Study the drawing (mm; zero at the part's minimum x, y, z) and answer. A direction names the side the tool comes from. Round coordinates to 2 decimals unless told otherwise and drop trailing zeros. Order: outer loops, then holes, each group sorted by start corner. A loop starts at its lowest first (then second) coordinate and runs counter-clockwise, first axis right, second up. Notation, with made-up numbers: (22.25, -23) - (66.25, -23) arc R23 cw to (66.25, -8) - close; hole circle Ø2 at (31, 48). An arc over 180 degrees is marked (long way). Use one line per item in the form item = value. Start each with the question number.
Q1. Which of the six approach directions +Z, -Z, +X, -X, +Y, -Y give full straight-line access (tool end or side, diameter ignored) to the marked faces 1 and 2?
Q2. For a pull along X with two mould halves and no side action, classify the marked faces 3, 4 and 5 as +X half, -X half, draft (parallel to the pull), parting line (faces both ways), or undercut.
Q3. The part is cut by section D-D on y = 14. Determine the outline of the cut face in (x, z) (1 decimal).
Q4. Given P1, Ø1, axis at y = 15, z = 0.5, coming from the -X side (1 decimal); P2, Ø1.5, axis at y = 15.5, z = 4.5, coming from the +X side; P3, Ø1.5, axis at x = 14, z = 1.5, coming from the -Y side (3 decimals), each flat-ended and moving along its own axis, determine where each tip first touches the part or whether it passes through.
Q5. Find the intervals of material crossed by line 1 (X direction, y = 16.5, z = 3); line 2 (X direction, y = 4.75, z = 0.75) (1 decimal); line 3 (Z direction, x = 4, y = 2.25), in increasing order. Write a range as [from, to].
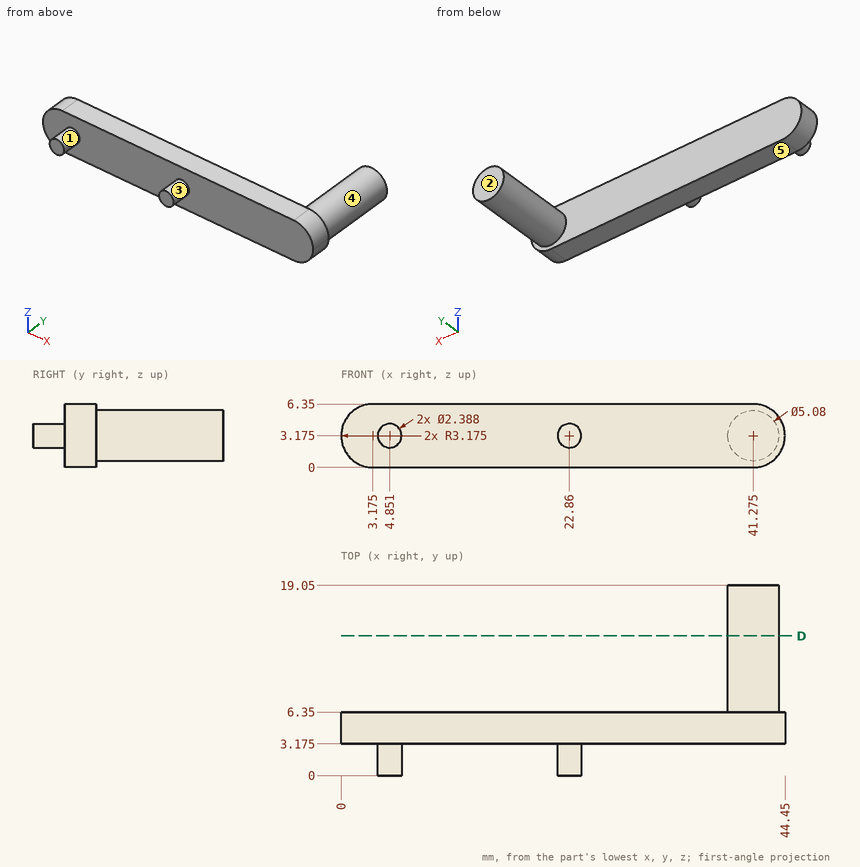
Found:
q1.face_1 = -Y
q1.face_2 = +Z, -Z, +X, -X, +Y
q2.face_3 = undercut
q2.face_4 = parting line
q2.face_5 = draft
q3.outline = circle Ø5.1 at (41.3, 3.2)
q4.P1 = 40
q4.P2 = 43.75
q4.P3 = 3.175
q5.line_1 = [38.74, 43.81]
q5.line_2 = [1.1, 43.3]
q5.line_3 = [2.34, 4.01]
